```python
from build123d import *

# Parameters (mm, degrees)
SKETCH1_W               = 38
SKETCH1_H               = 28
PCB_DEPTH               = 1.6
MOUNT_HOLE_1_DEPTH      = 48.22880477
MOUNT_HOLE_1_DEPTH_BACK = 48.22880477
SKETCH2_R               = 1.5
MOUNT_HOLE_2_DEPTH      = 48.22880477
MOUNT_HOLE_2_DEPTH_BACK = 48.22880477
SKETCH3_R               = 1.5
MOUNT_HOLE_3_DEPTH      = 48.22880477
MOUNT_HOLE_3_DEPTH_BACK = 48.22880477
SKETCH4_R               = 1.5
MOUNT_HOLE_4_DEPTH      = 48.22880477
MOUNT_HOLE_4_DEPTH_BACK = 48.22880477
SKETCH5_R               = 1.5
SENSOR_CONNECTOR_START  = 1.6
SKETCH6_W               = 7
SKETCH6_H               = 10
SENSOR_CONNECTOR_DEPTH  = 6
SIGNAL_CONNECTOR_START  = 1.6
SKETCH7_W               = 7
SKETCH7_H               = 10
SIGNAL_CONNECTOR_DEPTH  = 6
THRESHOLD_POT_START     = 1.6
SKETCH8_W               = 9.5
SKETCH8_H               = 9.5
THRESHOLD_POT_DEPTH     = 10
COMPARATOR_START        = 1.6
SKETCH9_W               = 5
SKETCH9_H               = 4
COMPARATOR_DEPTH        = 1.5


with BuildPart() as part:
    # Sketch1 → PCB (new body)
    with BuildSketch(Plane(origin=(0, 0, 0), x_dir=(1, 0, 0), z_dir=(0, 1, 0))):
        with Locations((19, 14)):
            Rectangle(SKETCH1_W, SKETCH1_H)
    extrude(amount=PCB_DEPTH)

    # Sketch2 → Mount_hole_1 (cut, two sides: drawn at the far end of the back side and taken through both)
    with BuildSketch(Plane(origin=(0, 0, 0), x_dir=(1, 0, 0), z_dir=(0, 1, 0)).offset(-MOUNT_HOLE_1_DEPTH_BACK)):
        with Locations(Location((3, 3, 0), (0, 0, 270))):
            Circle(SKETCH2_R)
    extrude(amount=MOUNT_HOLE_1_DEPTH + MOUNT_HOLE_1_DEPTH_BACK, mode=Mode.SUBTRACT)

    # Sketch3 → Mount_hole_2 (cut, two sides: drawn at the far end of the back side and taken through both)
    with BuildSketch(Plane(origin=(0, 0, 0), x_dir=(1, 0, 0), z_dir=(0, 1, 0)).offset(-MOUNT_HOLE_2_DEPTH_BACK)):
        with Locations(Location((35, 3, 0), (0, 0, 270))):
            Circle(SKETCH3_R)
    extrude(amount=MOUNT_HOLE_2_DEPTH + MOUNT_HOLE_2_DEPTH_BACK, mode=Mode.SUBTRACT)

    # Sketch4 → Mount_hole_3 (cut, two sides: drawn at the far end of the back side and taken through both)
    with BuildSketch(Plane(origin=(0, 0, 0), x_dir=(1, 0, 0), z_dir=(0, 1, 0)).offset(-MOUNT_HOLE_3_DEPTH_BACK)):
        with Locations(Location((3, 25, 0), (0, 0, 270))):
            Circle(SKETCH4_R)
    extrude(amount=MOUNT_HOLE_3_DEPTH + MOUNT_HOLE_3_DEPTH_BACK, mode=Mode.SUBTRACT)

    # Sketch5 → Mount_hole_4 (cut, two sides: drawn at the far end of the back side and taken through both)
    with BuildSketch(Plane(origin=(0, 0, 0), x_dir=(1, 0, 0), z_dir=(0, 1, 0)).offset(-MOUNT_HOLE_4_DEPTH_BACK)):
        with Locations(Location((35, 25, 0), (0, 0, 270))):
            Circle(SKETCH5_R)
    extrude(amount=MOUNT_HOLE_4_DEPTH + MOUNT_HOLE_4_DEPTH_BACK, mode=Mode.SUBTRACT)

    # Sketch6 → Sensor_connector (add)
    with BuildSketch(Plane(origin=(0, 0, 0), x_dir=(1, 0, 0), z_dir=(0, 1, 0)).offset(SENSOR_CONNECTOR_START)):
        with Locations((5.5, 14)):
            Rectangle(SKETCH6_W, SKETCH6_H)
    extrude(amount=SENSOR_CONNECTOR_DEPTH)

    # Sketch7 → Signal_connector (add)
    with BuildSketch(Plane(origin=(0, 0, 0), x_dir=(1, 0, 0), z_dir=(0, 1, 0)).offset(SIGNAL_CONNECTOR_START)):
        with Locations((32.5, 14)):
            Rectangle(SKETCH7_W, SKETCH7_H)
    extrude(amount=SIGNAL_CONNECTOR_DEPTH)

    # Sketch8 → Threshold_pot (add)
    with BuildSketch(Plane(origin=(0, 0, 0), x_dir=(1, 0, 0), z_dir=(0, 1, 0)).offset(THRESHOLD_POT_START)):
        with Locations((19.75, 8.75)):
            Rectangle(SKETCH8_W, SKETCH8_H)
    extrude(amount=THRESHOLD_POT_DEPTH)

    # Sketch9 → Comparator (add)
    with BuildSketch(Plane(origin=(0, 0, 0), x_dir=(1, 0, 0), z_dir=(0, 1, 0)).offset(COMPARATOR_START)):
        with Locations((18.5, 19)):
            Rectangle(SKETCH9_W, SKETCH9_H)
    extrude(amount=COMPARATOR_DEPTH)


solid = part.part
```
CAD build for the part. Positions are in the model's coordinates, mm. A direction names the side the tool comes from. Give positions to 0.01 mm unless a question says otherwise; leave off trailing zeros. Write each loop counter-clockwise with the first axis right and the second up, starting at its lowest first coordinate (ties: lowest second). Pieces come first, ordered by that corner, then holes. Notation, with made-up numbers: M 33,22 L 49,22 A30 ccw 49,53 Z; hole C 27,-11 d11. An arc over 180 degrees is marked long. Return JSON: item names as keys, results as strings. Group by question number.
(1) Flat gauge pins, fed straight in: pin 1 Ø6 at (x, y) = (27.5, 7) entering from -Z; pin 2 Ø1.8 at (y, z) = (5, -12) entering from -X; pin 3 Ø3 at (x, z) = (9.5, -7.5) entering from +Y. Where does each tip first touch, or does it go through?
(2) Band-saw the part on B-B (y = 6). Give the cut face in (x, z).
(3) Band-saw the part on A-A (x = 35). Give the cut face in (y, z).
(4) Band-saw the part on C-C (z = -3). Give the cut face in (x, y), and give its area (3 significant figures).
(5) 3-axis set-ups, long thin cutter, end or side, ignore diameter. For faces 4 (the face through (24.5, 7, -9)), 5 (the face through (36, 5, -14)), 6 (the face through (18, 3.1, -19)), 7 (the face through (32, 5, -19)), 8 (the face through (20, 7, -4)): which of +Z, -Z, +X, -X, +Y, -Y reach the whole face in a straight line?
(6) Mould opens along X. For faces 1 (the face through (3.07, 0.79, -26.5)), 2 (the face through (2, 5, -14)), 3 (the face through (5, 7.6, -14)) say: pulls with the +X half, pulls with the -X half, needs draft (parallel to the pull), parting line crosses it, or undercut.
(7) Drill centre lines: L1, parallel to Z at x = 3, y = 0.7; L2, parallel to X at y = 1.35, z = -3; L3, parallel to Z at x = 33.5, y = 6.5. Where is each one in solid material? Low to high. Write a range as [from, to].
(8) Band-saw the part on D-D (z = -15.75). Give the cut face in (x, y).
Entries:
{
 "1": {"pin 1": "stops at z = -19", "pin 2": "stops at x = 2", "pin 3": "stops at y = 1.6"},
 "2": {"outline": "M 2,-19 L 9,-19 L 9,-9 L 2,-9 Z; M 15,-13.5 L 24.5,-13.5 L 24.5,-4 L 15,-4 Z; M 29,-19 L 36,-19 L 36,-9 L 29,-9 Z"},
 "3": {"outline": "M 0,-28 L 1.6,-28 L 1.6,-26.5 L 0,-26.5 Z; M 0,-23.5 L 1.6,-23.5 L 1.6,-19 L 7.6,-19 L 7.6,-9 L 1.6,-9 L 1.6,-4.5 L 0,-4.5 Z; M 0,-1.5 L 1.6,-1.5 L 1.6,0 L 0,0 Z"},
 "4": {"outline": "M 0,0 L 1.5,0 L 1.5,1.6 L 0,1.6 Z; M 4.5,0 L 33.5,0 L 33.5,1.6 L 4.5,1.6 Z; M 36.5,0 L 38,0 L 38,1.6 L 36.5,1.6 Z", "area": "51.2 mm^2"},
 "5": {"face 4": "+Z, -Z, +Y", "face 5": "+Z, -Z, +X, +Y", "face 6": "-Z, +Y", "face 7": "-Z, +X, +Y", "face 8": "+Z, +X, -X, +Y"},
 "6": {"face 1": "undercut", "face 2": "pulls with the -X half", "face 3": "needs draft"},
 "7": {"L1": "z = [-28, -26.5], [-23.5, -4.5], [-1.5, 0]", "L2": "x = [0, 1.5], [4.5, 33.5], [36.5, 38]", "L3": "z = [-19, -9]"},
 "8": {"outline": "M 0,0 L 38,0 L 38,1.6 L 36,1.6 L 36,7.6 L 29,7.6 L 29,1.6 L 9,1.6 L 9,7.6 L 2,7.6 L 2,1.6 L 0,1.6 Z"}
}
